Geometry: see drawing. Coordinates: mm, zero at the bounding-box minimum. Round coordinates to 2 decimals unless told otherwise and drop trailing zeros. Write each loop counter-clockwise with the first axis right and the second up, starting at its lowest first coordinate (ties: lowest second). Pieces come first, ordered by that corner, then holes. Notation, with made-up numbers: M -3.5,55.25 L 37.5,55.25 A26 cw 37.5,81.25 Z; hole C -13,13 d8. An arc over 180 degrees is marked long. Use a Markdown table: item, result.
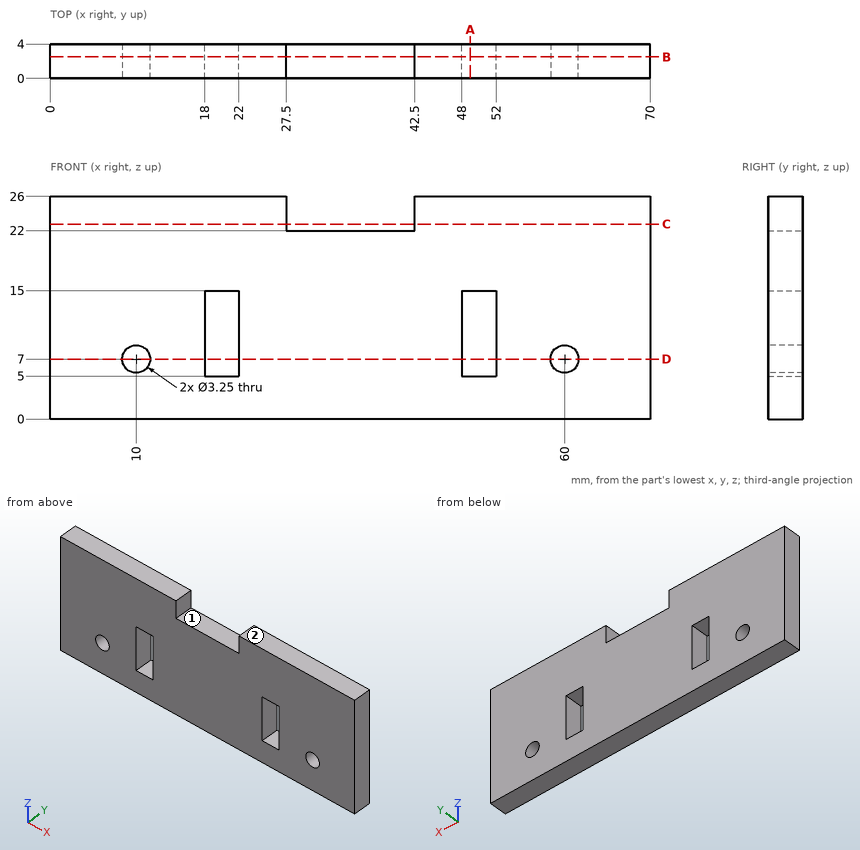
Q1. Line query: L1, parallel to X at y = 2, z = 13.75; L2, parallel to X at y = 0.9, z = 7 (3 decimals); L3, parallel to Z at x = 60, y = 1.9 (3 decimals). Output: solid intervals per line, ascending.
Results are:
| item | result |
|---|---|
| L1 | 0 to 18, 22 to 48, 52 to 70 |
| L2 | 0 to 8.375, 11.625 to 18, 22 to 48, 52 to 58.375, 61.625 to 70 |
| L3 | 0 to 5.375, 8.625 to 26 |
Q2. Section D-D on z = 7. Return loops of the section in (x, y) (3 decimals).
Results are:
| item | result |
|---|---|
| outline | M 0,0 L 8.375,0 L 8.375,4 L 0,4 Z; M 11.625,0 L 18,0 L 18,4 L 11.625,4 Z; M 22,0 L 48,0 L 48,4 L 22,4 Z; M 52,0 L 58.375,0 L 58.375,4 L 52,4 Z; M 61.625,0 L 70,0 L 70,4 L 61.625,4 Z |
Q3. First-contact query: pin 1 Ø1.9 at (x, z) = (60, 7) entering from +Y; pin 2 Ø2 at (x, y) = (35.5, 1.5) entering from +Z. Flat tips, straight axial feed; report the tip coordinate or a pass-through.
Results are:
| item | result |
|---|---|
| pin 1 | through |
| pin 2 | z = 22 |
Q4. Section A-A on x = 49. Return loops of the section in (y, z).
Results are:
| item | result |
|---|---|
| outline | M 0,0 L 4,0 L 4,5 L 0,5 Z; M 0,15 L 4,15 L 4,26 L 0,26 Z |
Q5. Section B-B on y = 2.5. Return loops of the section in (x, z) (3 decimals), plus the area to 3 significant figures.
Results are:
| item | result |
|---|---|
| outline | M 0,0 L 70,0 L 70,26 L 42.5,26 L 42.5,22 L 27.5,22 L 27.5,26 L 0,26 Z; hole C 10,7 d3.25; hole M 18,5 L 22,5 L 22,15 L 18,15 Z; hole M 48,5 L 52,5 L 52,15 L 48,15 Z; hole C 60,7 d3.25 |
| area | 1,660 mm^2 |
Q6. Mould query, pull axis X, two halves, no side actions, for the marked faces 1 and 2. Classes: +X half, -X half, draft (parallel to the pull), parting line (faces both ways), or undercut.
Results are:
| item | result |
|---|---|
| face 1 | undercut |
| face 2 | draft |
Q7. Section C-C on z = 22.75. Return loops of the section in (x, y), plus the area to 3 significant figures.
Results are:
| item | result |
|---|---|
| outline | M 0,0 L 27.5,0 L 27.5,4 L 0,4 Z; M 42.5,0 L 70,0 L 70,4 L 42.5,4 Z |
| area | 220 mm^2 |
